Design review of the part shown in the three views and the two pictorial views. Dimensions are in mm from the part's minimum x, y and z. Give positions to 0.01 mm unless a question says otherwise; leave off trailing zeros. Order: outer loops, then holes, each group sorted by start corner. A loop starts at its lowest first (then second) coordinate and runs counter-clockwise, first axis right, second up.
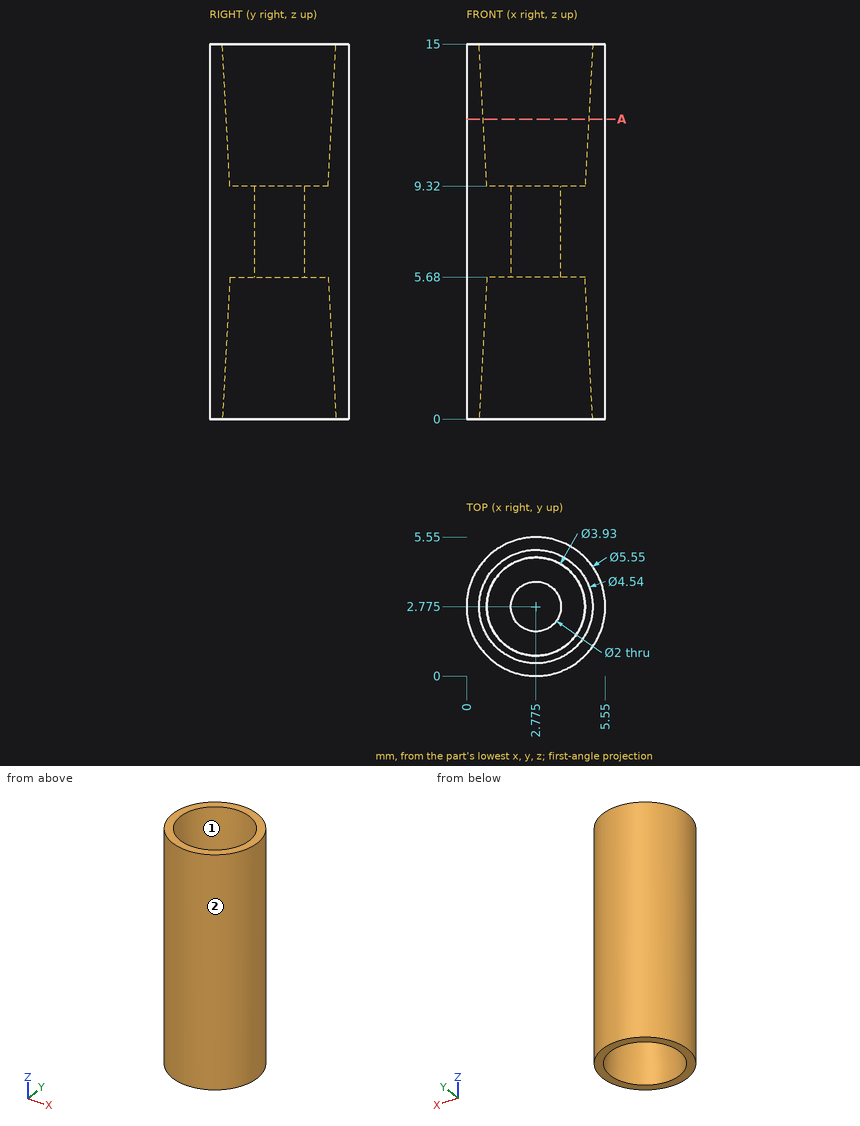
1) To check wall thickness, follow line 1 (Y direction, x = 2.5, z = 11); line 2 (X direction, y = 2.55, z = 12.75); line 3 (Z direction, x = 2.55, y = 4.1). State the ranges of each line that lie inside material, in increasing order.
Answer sheet:
line 1: y = 0.01 to 0.74, 4.81 to 5.54
line 2: x = 0.01 to 0.64, 4.91 to 5.54
line 3: z = 5.68 to 9.32
2) Clearance check with flat-ended pins moving along their axes: pin 1 (2 mm diameter, centred on x = 1.5, z = 9, fed in from +Y); pin 2 (2 mm diameter, centred on x = 4, z = 4, fed in from -Y); pin 3 (2 mm diameter, centred on x = 2.5, y = 2, fed in from +Z). State where each tip first meets the part, or that it passes through.
Answer sheet:
pin 1: stops at y = 5.54
pin 2: stops at y = 0.01
pin 3: stops at z = 9.32
3) Draft analysis for pull direction X (two halves, no side actions). For the marked faces 1 and 2, state which applies: +X half, -X half, draft (parallel to the pull), parting line (faces both ways), or undercut.
Answer sheet:
face 1: undercut
face 2: parting line
4) We need section A-A on z = 12. Give the boundary of the cut face in (x, y) (3 decimals).
Answer sheet:
outline: circle Ø5.55 at (2.775, 2.775); hole circle Ø4.218 at (2.775, 2.775)
